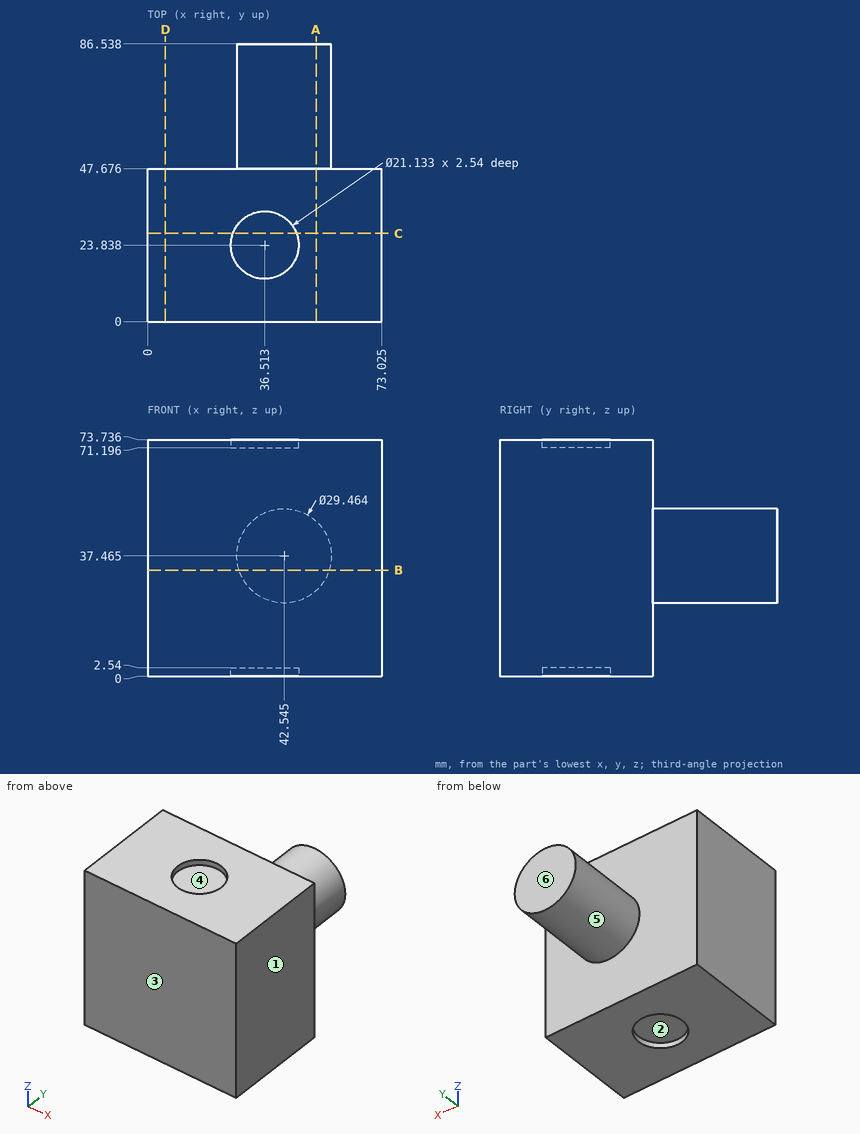
Could you check a few things on this drawing? It's one solid part, dimensions in mm from its lowest x, y, z. A direction names the side the tool comes from. Give positions to 0.01 mm unless a question says otherwise; leave off trailing zeros. Write each loop counter-clockwise with the first axis right and the second up, starting at its lowest first coordinate (ties: lowest second). Pieces come first, ordered by that corner, then holes. Notation, with made-up numbers: (-30.5, 49) -> (22.5, 49) arc R25 ccw to (22.5, 64) -> close; hole circle Ø7 at (29, 33). An arc over 180 degrees is marked (long way). Answer as CSV lines item,"result". Start each with the question number.
(1) Please list where these lines run through material, in increasing order: line 1 (Y direction, x = 54, z = 60) (1 decimal); line 2 (Z direction, x = 43, y = 75.5); line 3 (X direction, y = 77, z = 37).
(2) Which directions (+Z, -Z, +X, -X, +Y, -Y) give clear straight access to the entire face, cutting with the end or side of a thin tool? Please do the marked faces 4, 5 and 6.
(3) If we section it at D-D, the plane x = 5.5: Write out the boundary of the cut face in (y, z) (1 decimal), and give its area (3 significant figures).
(4) If we section it at B-B, the plane z = 33: Write out the boundary of the cut face in (x, y) (1 decimal), and give its area (3 significant figures).
(5) If we section it at A-A, the plane x = 52.5: Write out the boundary of the cut face in (y, z) (1 decimal).
(6) If we section it at C-C, the plane y = 27.5: Write out the boundary of the cut face in (x, z) (1 decimal).
(7) If we mould it in two halves opening along Y, with no side actions, what happens to the marked faces 1, 2 and 3? For each: +Y half, -Y half, draft (parallel to the pull), parting line (faces both ways), or undercut.
(8) I'm going to push flat-ended pins straight in: pin 1 Ø10.5 at (x, y) = (40.5, 20) entering from +Z; pin 2 Ø8 at (x, y) = (8.5, 55) entering from +Z; pin 3 Ø8 at (x, y) = (47, 72.5) entering from +Z; pin 4 Ø6.5 at (x, y) = (35.5, 25.5) entering from -Z. Where does each tip first touch, or does it pass through?
Answer list:
1,line 1,"0 to 47.7"
1,line 2,"22.74 to 52.19"
1,line 3,"27.82 to 57.27"
2,face 4,"+Z"
2,face 5,"+Y"
2,face 6,"+Z, -Z, +X, -X, +Y"
3,outline,"(0, 0) -> (47.7, 0) -> (47.7, 73.7) -> (0, 73.7) -> close"
3,area,"3,520 mm^2"
4,outline,"(0, 0) -> (73, 0) -> (73, 47.7) -> (56.6, 47.7) -> (56.6, 86.5) -> (28.5, 86.5) -> (28.5, 47.7) -> (0, 47.7) -> close"
4,area,"4,570 mm^2"
5,outline,"(0, 0) -> (47.7, 0) -> (47.7, 26.6) -> (86.5, 26.6) -> (86.5, 48.3) -> (47.7, 48.3) -> (47.7, 73.7) -> (0, 73.7) -> close"
6,outline,"(0, 0) -> (26.6, 0) -> (26.6, 2.5) -> (46.4, 2.5) -> (46.4, 0) -> (73, 0) -> (73, 73.7) -> (46.4, 73.7) -> (46.4, 71.2) -> (26.6, 71.2) -> (26.6, 73.7) -> (0, 73.7) -> close"
7,face 1,"draft"
7,face 2,"undercut"
7,face 3,"-Y half"
8,pin 1,"z = 73.74"
8,pin 2,"through"
8,pin 3,"z = 52.19"
8,pin 4,"z = 2.54"
